Can you work these out from the drawing? Everything is in mm from the part's minimum corner. A direction names the side the tool comes from. Round coordinates to 2 decimals unless told otherwise and drop trailing zeros. Write each loop counter-clockwise with the first axis right and the second up, starting at its lowest first coordinate (ties: lowest second). Pieces come first, ordered by that corner, then holes. Notation, with made-up numbers: (75, 78.5) - (97, 78.5) arc R19 ccw to (97, 115.5) - close; hole circle Ø7 at (63.5, 32). An arc over 180 degrees is marked (long way). Write each question's results on one line, items separated by ' | '. Start each with the question number.
(1) Imagine slicing it at C-C on x = 10.5. Write out the boundary of the cut face in (y, z).
(2) Imagine slicing it at A-A on z = 7.5. Write out the boundary of the cut face in (x, y), then the cut area to 3 significant figures.
(3) Imagine slicing it at B-B on y = 25.5. Write out the boundary of the cut face in (x, z), then the cut area to 3 significant figures.
(4) Thinking about a two-plate mould opening in X: for the marked faces 1, 2 and 3, which applies, +X half, -X half, draft (parallel to the pull), parting line (faces both ways), or undercut?
(5) On a 3-axis mill with a long thin cutter (end or side, diameter ignored), from which of +Z, -Z, +X, -X, +Y, -Y can I reach the whole of each face in a straight line? I mean the marked faces 4, 5, 6 and 7. Say none if no direction works.
(6) Please list where these lines run through material, in increasing order: line 1 (X direction, y = 25.75, z = 4.5); line 2 (Z direction, x = 7, y = 16.75); line 3 (Y direction, x = 10.75, z = 4.5). Write a range as [from, to].
(7) Imagine slicing it at D-D on y = 9. Write out the boundary of the cut face in (x, z), then the cut area to 3 significant figures.
(8) For P1, Ø0.6, axis at x = 0.5, z = 4, coming from the -Y side; P2, Ø3, axis at x = 3, z = 6.5, coming from the -Y side; P3, Ø1.9, axis at y = 16, z = 6, coming from the +X side, each with a flat end and sliding along its axis, tell me the tip position at first contact or that it passes through.
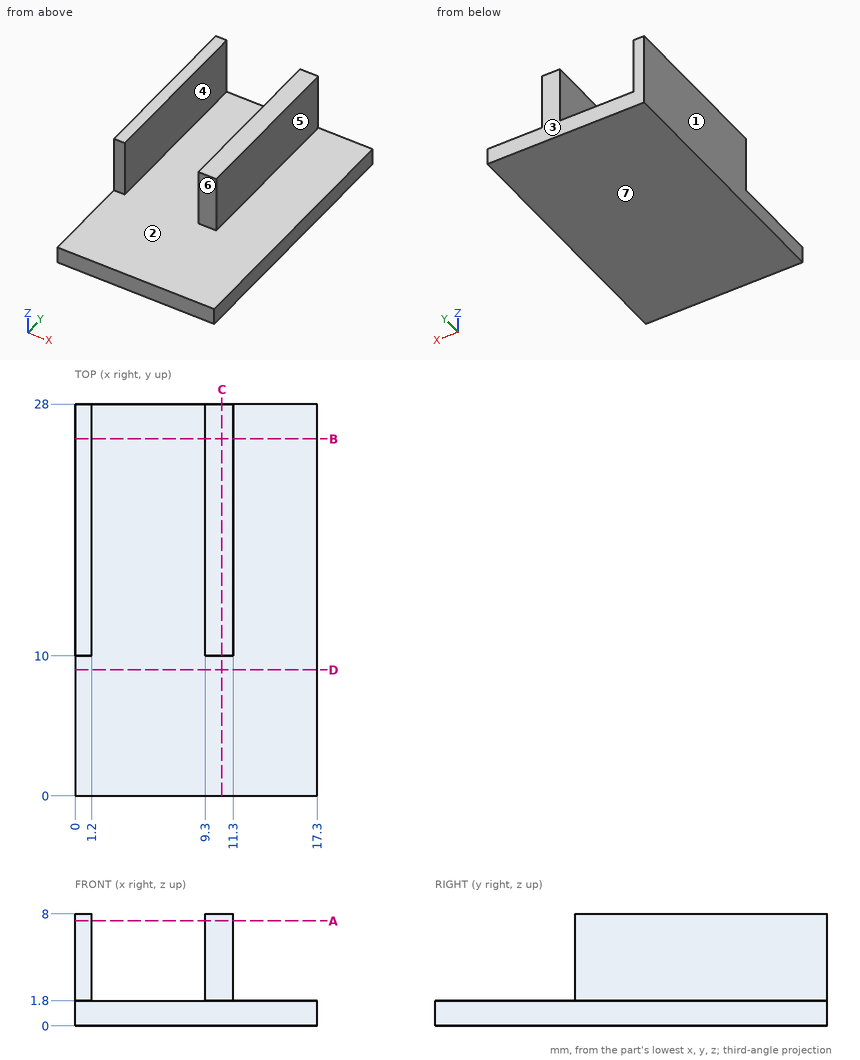
Response:
1) outline: (0, 0) - (28, 0) - (28, 8) - (10, 8) - (10, 1.8) - (0, 1.8) - close
2) outline: (0, 10) - (1.2, 10) - (1.2, 28) - (0, 28) - close; (9.3, 10) - (11.3, 10) - (11.3, 28) - (9.3, 28) - close | area: 57.6 mm²
3) outline: (0, 0) - (17.3, 0) - (17.3, 1.8) - (11.3, 1.8) - (11.3, 8) - (9.3, 8) - (9.3, 1.8) - (1.2, 1.8) - (1.2, 8) - (0, 8) - close | area: 51.0 mm²
4) face 1: -X half | face 2: undercut | face 3: draft
5) face 4: +Z, +Y, -Y | face 5: +Z, +X, +Y, -Y | face 6: +Z, +X, -X, -Y | face 7: -Z, +X, -X, +Y, -Y
6) line 1: [0, 1.2], [9.3, 11.3] | line 2: [0, 1.8] | line 3: [10, 28]
7) outline: (0, 0) - (17.3, 0) - (17.3, 1.8) - (0, 1.8) - close | area: 31.1 mm²
8) P1: y = 10 | P2: through | P3: x = 11.3
